```python
from build123d import *

# Parameters (mm, degrees)
BOSS_EXTRUDE1_DEPTH = 20
SKETCH2_W           = 30
SKETCH2_H           = 6
BOSS_EXTRUDE2_DEPTH = 3
SKETCH3_W           = 50
SKETCH3_H           = 3
BOSS_EXTRUDE3_DEPTH = 6
SKETCH4_W           = 3
SKETCH4_H           = 6
BOSS_EXTRUDE4_DEPTH = 6.5


with BuildPart() as part:
    # Sketch1 → Boss-Extrude1 (new body)
    with BuildSketch(Plane(origin=(0, 0, 0), x_dir=(0, 0, -1), z_dir=(1, 0, 0))):
        Polygon((-9.8, -6.5), (-3.8, -6.5), (-3.8, -3.357082066), (0, 0), (-5.1, 0), (-5.1, 37.85), (-0.3, 37.85), (-0.3, 41), (-9.8, 41), align=None)
    extrude(amount=BOSS_EXTRUDE1_DEPTH)

    # Sketch2 → Boss-Extrude2 (add)
    with BuildSketch(Plane.XZ.offset(6.5)):
        with Locations((10, 6.8)):
            Rectangle(SKETCH2_W, SKETCH2_H)
    extrude(amount=-BOSS_EXTRUDE2_DEPTH)

    # Sketch3 → Boss-Extrude3 (add)
    with BuildSketch(Plane(origin=(0, 0, 3.8), x_dir=(-1, 0, 0), z_dir=(0, 0, -1))):
        with Locations((-10, -5)):
            Rectangle(SKETCH3_W, SKETCH3_H)
    extrude(amount=-BOSS_EXTRUDE3_DEPTH)

    # Sketch4 → Boss-Extrude4 (add)
    with BuildSketch(Plane.XZ.offset(6.5)):
        with Locations((-13.5, 6.8)):
            Rectangle(SKETCH4_W, SKETCH4_H)
        with Locations((33.5, 6.8)):
            Rectangle(SKETCH4_W, SKETCH4_H)
    extrude(amount=BOSS_EXTRUDE4_DEPTH)


solid = part.part
```
Here's how the part is built. I have some questions about the finished solid (model axes, mm). A direction names the side the tool comes from. Give positions to 0.01 mm unless a question says otherwise; leave off trailing zeros. Order: outer loops, then holes, each group sorted by start corner. A loop starts at its lowest first (then second) coordinate and runs counter-clockwise, first axis right, second up. Notation, with made-up numbers: M -35,15.25 L -29,15.25 A15 cw -29,38.25 Z; hole C 49.5,18.5 d9. An arc over 180 degrees is marked long. Use a Markdown table: item, result. Add a question column.
1. If we mould it in two halves opening along Y, with no side actions, what happens to faces 1 (the flat face through (-14, -13, 7)), 2 (the flat face through (10, 0, 3)), 3 (the flat face through (10, 39, 0.3)), 4 (the flat face through (10, 19, 5.1))? For each: +Y half, -Y half, draft (parallel to the pull), parting line (faces both ways), or undercut.
2. Suppose I cut it at B-B (x = 13.5). List the corners of the cut face in (y, z) for me.
3. Suppose I cut it at A-A (z = 4.5). List the corners of the cut face in (x, y) for me, and give its area (3 significant figures).
4. Suppose I cut it at D-D (y = -5.5). List the corners of the cut face in (x, z) for me, and give its area (3 significant figures).
5. I need wall thicknesses on probe 1 along Y at (x, z) = (21.5, 6.5); probe 2 along Y at (x, z) = (7, 8); probe 3 along Z at (x, y) = (16, 23.5). Which ranges of each line are inside material? Lowest first, please. Write a range as from..to.
6. Suppose I cut it at C-C (y = 34.5). List the corners of the cut face in (x, z) for me.
7. For pin 1 Ø3 at (y, z) = (18, 3.5) entering from -X; pin 2 Ø5 at (x, z) = (-9.5, 6.5) entering from +Y; pin 3 Ø5 at (y, z) = (5.5, 8) entering from +X; pin 4 Ø7.5 at (x, y) = (6, -7) entering from -Z, each with a flat end and sliding along its axis, tell me the tip position at first contact or that it passes through.
8. On a 3-axis mill with a long thin cutter (end or side, diameter ignored), from which of +Z, -Z, +X, -X, +Y, -Y can I reach the whole of each face in a straight line? I mean faces 5 (the flat face through (10, 37.85, 3)), 6 (the flat face through (4, -6, 3.8)), 7 (the flat face through (10, -6.5, 7)), 8 (the flat face through (-8, -3.5, 7)), 9 (the flat face through (20, 19, 7)). Say none if no direction works.
Results list:
| question | item | result |
|---|---|---|
| 1 | face 1 | -Y half |
| 1 | face 2 | undercut |
| 1 | face 3 | draft |
| 1 | face 4 | undercut |
| 2 | outline | M -6.5,3.8 L -3.36,3.8 L 0,0 L 0,5.1 L 37.85,5.1 L 37.85,0.3 L 41,0.3 L 41,9.8 L -6.5,9.8 Z |
| 3 | outline | M -15,-13 L -12,-13 L -12,-6.5 L 32,-6.5 L 32,-13 L 35,-13 L 35,-3.5 L 20,-3.5 L 20,0 L 0,0 L 0,-3.5 L -15,-3.5 Z; M 0,37.85 L 20,37.85 L 20,41 L 0,41 Z |
| 3 | area | 322 mm² |
| 4 | outline | M -15,3.8 L 35,3.8 L 35,9.8 L -15,9.8 Z |
| 4 | area | 300 mm² |
| 5 | probe 1 | y = -6.5..-3.5 |
| 5 | probe 2 | y = -6.5..41 |
| 5 | probe 3 | z = 5.1..9.8 |
| 6 | outline | M 0,5.1 L 20,5.1 L 20,9.8 L 0,9.8 Z |
| 7 | pin 1 | passes through |
| 7 | pin 2 | stops at y = -3.5 |
| 7 | pin 3 | stops at x = 20 |
| 7 | pin 4 | stops at z = 3.68 |
| 8 | face 5 | -Z, +X, -X |
| 8 | face 6 | -Z, +X, -X, -Y |
| 8 | face 7 | +Z, -Z, -Y |
| 8 | face 8 | +Z, -Z, -X, +Y |
| 8 | face 9 | +Z, -Z, +X, +Y |
